Input: part model. Units: mm. Frame: model coordinates. Face numbers are marked on the shaded views. A direction names the side the tool comes from. Give positions to 0.01 mm unless a question says otherwise; leave off trailing zeros. Loops run counter-clockwise (first coordinate to the right, second up) from the corner with the lowest first, then second, coordinate; pieces in that order, holes last. Notation, with made-up numbers: (60.5, 22.5) - (78.5, 22.5) arc R11 cw to (78.5, 33.5) - close; hole circle Ø5 at (63, 60). An arc over 180 degrees is marked (long way). Answer as a JSON object with one key per item and string values.
Autodesk Fusion 360 part; units mm, degrees
sketch "Sketch1" plane through (0, 0, 0) normal (0, 0, 1) x (1, 0, 0) in component "Component"
  line L0 (0, 0) -> (63.5, 0)
  line L1 (63.5, 0) -> (63.5, 19.05)
  line L2 (63.5, 19.05) -> (19.05, 19.05)
  line L3 (19.05, 19.05) -> (19.05, 63.5)
  line L4 (19.05, 63.5) -> (0, 63.5)
  line L5 (0, 63.5) -> (0, 0)
  dimension "d1" = 63.5
  dimension "d2" = 63.5
  dimension "d3" = 19.05
  dimension "d4" = 19.05
extrude "Extrude1" add sketch "Sketch1" along normal blind 63.5 in component "Component"
sketch "Sketch2" plane through (0, 63.5, 0) normal (0, 1, 0) x (-1, 0, 0) in component "Component"
  line L0 (-19.05, 0) -> (0, 0)
  line L1 (0, 0) -> (0, 63.5)
  line L2 (0, 63.5) -> (-19.05, 63.5)
  line L3 (-19.05, 63.5) -> (-19.05, 0)
  line L4 (0, 0) -> (63.5, 0)
  line L5 (63.5, 0) -> (63.5, 63.5)
  line L6 (63.5, 63.5) -> (44.45, 63.5)
  line L7 (44.45, 63.5) -> (44.45, 19.05)
  line L8 (44.45, 19.05) -> (0, 19.05)
  line L9 (0, 19.05) -> (0, 0)
  dimension "d7" = 63.5
  dimension "d8" = 63.5
  dimension "d9" = 19.05
  dimension "d10" = 19.05
extrude "Extrude2" add sketch "Sketch2" against normal blind 63.5 contours L1 L4 L5 L6 L7 L8 L9 in component "Component"
sketch "Sketch3" plane through (0, 19.05, 0) normal (0, 1, 0) x (-1, 0, 0) in component "Component"
  line L0 (-63.5, 0) -> (-19.05, 0)
  line L1 (-19.05, 0) -> (-19.05, 63.5)
  line L2 (-19.05, 63.5) -> (-63.5, 63.5)
  line L3 (-63.5, 63.5) -> (-63.5, 0)
  circle A0 centre (-44.45, 31.75) radius 9.525
  dimension "d13" = 19.05
  dimension "d14" = 31.75
  dimension "d15" = 19.05
extrude "Extrude3" cut sketch "Sketch3" against normal through all contours A0 in component "Component"
sketch "Sketch4" plane through (19.05, 0, 0) normal (1, 0, 0) x (0, 1, 0) in component "Component"
  line L0 (19.05, 0) -> (63.5, 0)
  line L1 (63.5, 0) -> (63.5, 63.5)
  line L2 (63.5, 63.5) -> (19.05, 63.5)
  line L3 (19.05, 63.5) -> (19.05, 0)
  line L4 (63.5, 38.1) -> (38.1, 63.5)
  dimension "d17" = 25.4
  dimension "d18" = 45
extrude "Extrude4" cut sketch "Sketch4" against normal up to surface (19.05 mm away) contours L1 L2 L4 in component "Component"
component "Component" placed x (1, 0, 0) y (0, 1, 0) z (0, 0, 1) at (0, 0, 0)
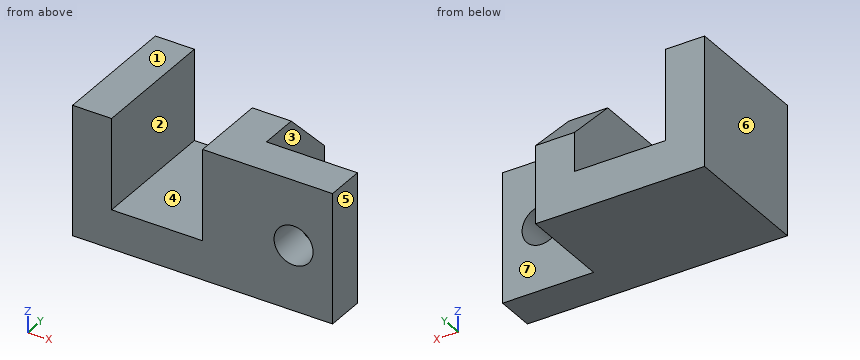
Item 1: Contact query for flat-ended pins moving along their axis: P1, Ø2, axis at x = 49, z = 53, coming from the +Y side; P2, Ø12, axis at x = 27.5, z = 9, coming from the -Y side; P3, Ø13.5, axis at y = 43, z = 48.5, coming from the +X side; P4, Ø13.5, axis at x = -29, y = 47.5, coming from the +Z side. Output: stop coordinate, or through.
Geometry check:
{"P1": "stops at y = 19.05", "P2": "stops at y = 0", "P3": "stops at x = 19.05", "P4": "stops at z = 19.05"}
Item 2: Cut plane D-D (y = 42). Return loops of the section in (x, z), then the cut area to 3 significant figures.
Geometry check:
{"outline": "(-63.5, 0) - (19.05, 0) - (19.05, 59.6) - (0, 59.6) - (0, 19.05) - (-44.45, 19.05) - (-44.45, 63.5) - (-63.5, 63.5) - close", "area": "3,190 mm2"}
Item 3: Cut plane A-A (y = 12). Return loops of the section in (x, z) (3 decimals), then the cut area to 3 significant figures.
Geometry check:
{"outline": "(-63.5, 0) - (63.5, 0) - (63.5, 63.5) - (0, 63.5) - (0, 19.05) - (-44.45, 19.05) - (-44.45, 63.5) - (-63.5, 63.5) - close; hole circle Ø19.05 at (44.45, 31.75)", "area": "5,800 mm2"}
Item 4: Cut plane B-B (x = 44.45). Return loops of the section in (y, z) (3 decimals), then the cut area to 3 significant figures.
Geometry check:
{"outline": "(0, 0) - (19.05, 0) - (19.05, 22.225) - (0, 22.225) - close; (0, 41.275) - (19.05, 41.275) - (19.05, 63.5) - (0, 63.5) - close", "area": "847 mm2"}
Item 5: Cut plane C-C (z = 31.75). Return loops of the section in (x, y) (3 decimals), then the cut area to 3 significant figures.
Geometry check:
{"outline": "(-63.5, 0) - (-44.45, 0) - (-44.45, 63.5) - (-63.5, 63.5) - close; (0, 0) - (34.925, 0) - (34.925, 19.05) - (19.05, 19.05) - (19.05, 63.5) - (0, 63.5) - close; (53.975, 0) - (63.5, 0) - (63.5, 19.05) - (53.975, 19.05) - close", "area": "2,900 mm2"}
Item 6: Mould query, pull axis X, two halves, no side actions, for the marked faces 4, 5, 6 and 7. Classes: released by +X, released by -X, zero draft, split by the parting line, or undercut.
Geometry check:
{"face 4": "undercut", "face 5": "released by +X", "face 6": "released by -X", "face 7": "zero draft"}
Item 7: Material intervals for line 1 (X direction, y = 4.5, z = 53); line 2 (Z direction, x = 44.45, y = 14) (3 decimals); line 3 (X direction, y = 45, z = 53.5), sorted ascending. Write a range as [from, to].
Geometry check:
{"line 1": "x = [-63.5, -44.45], [0, 63.5]", "line 2": "z = [0, 22.225], [41.275, 63.5]", "line 3": "x = [-63.5, -44.45], [0, 19.05]"}
Item 8: Access query for the marked faces 1, 2 and 3. Directions: +Z, -Z, +X, -X, +Y, -Y. A direction counts if a zero-diameter tool reaches every point of the face in a straight line with its end or side. Return the directions, or none.
Geometry check:
{"face 1": "+Z, +X, -X, +Y, -Y", "face 2": "+Z, +Y, -Y", "face 3": "+Z, -Z, +X, +Y"}
